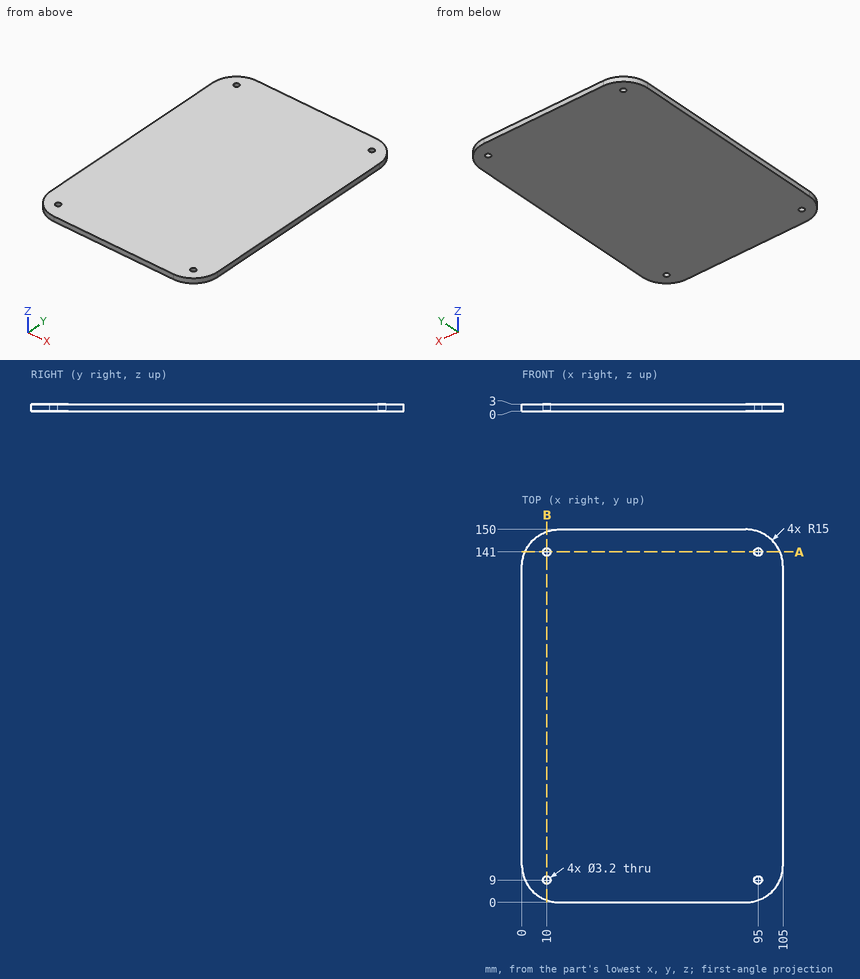
Job drawing, mm, ordinate dimensions from the low corner. One solid piece. Coordinates: 2 decimals unless noted, no trailing zeros. Order: outer loops, then holes, each group sorted by start corner. A loop starts at its lowest first (then second) coordinate and runs counter-clockwise, first axis right, second up. Notation, with made-up numbers: (-2.75, 87) - (40.25, 87) arc R28 ccw to (40.25, 124) - close; hole circle Ø9 at (63.25, 71.25). An arc over 180 degrees is marked (long way). Write each question's results on one line, items separated by ' | '. Start each with the question number.
Item 1: Band-saw the part on B-B on x = 10. Write the cut outline in (y, z), and give its area (3 significant figures).
Item 2: Wall check: probe 1 along Y at (x, z) = (10, 0.8); probe 2 along X at (y, z) = (141, 1.3); probe 3 along X at (y, z) = (137, 0.6). Give the ranges that are in metal, low to high. Write a range as [from, to].
Item 3: Flat gauge pin, fed straight in: pin 1 (1.9 mm diameter, centred on x = 10, y = 9, fed in from -Z). Where does the tip first touch, or does it go through?
Item 4: Band-saw the part on A-A on y = 141. Write the cut outline in (x, z).
Numbers:
1) outline: (0.86, 0) - (7.4, 0) - (7.4, 3) - (0.86, 3) - close; (10.6, 0) - (139.4, 0) - (139.4, 3) - (10.6, 3) - close; (142.6, 0) - (149.14, 0) - (149.14, 3) - (142.6, 3) - close | area: 426 mm^2
2) probe 1: [0.86, 7.4], [10.6, 139.4], [142.6, 149.14] | probe 2: [1.25, 8.4], [11.6, 93.4], [96.6, 103.75] | probe 3: [0.13, 104.87]
3) pin 1: through
4) outline: (1.25, 0) - (8.4, 0) - (8.4, 3) - (1.25, 3) - close; (11.6, 0) - (93.4, 0) - (93.4, 3) - (11.6, 3) - close; (96.6, 0) - (103.75, 0) - (103.75, 3) - (96.6, 3) - close
